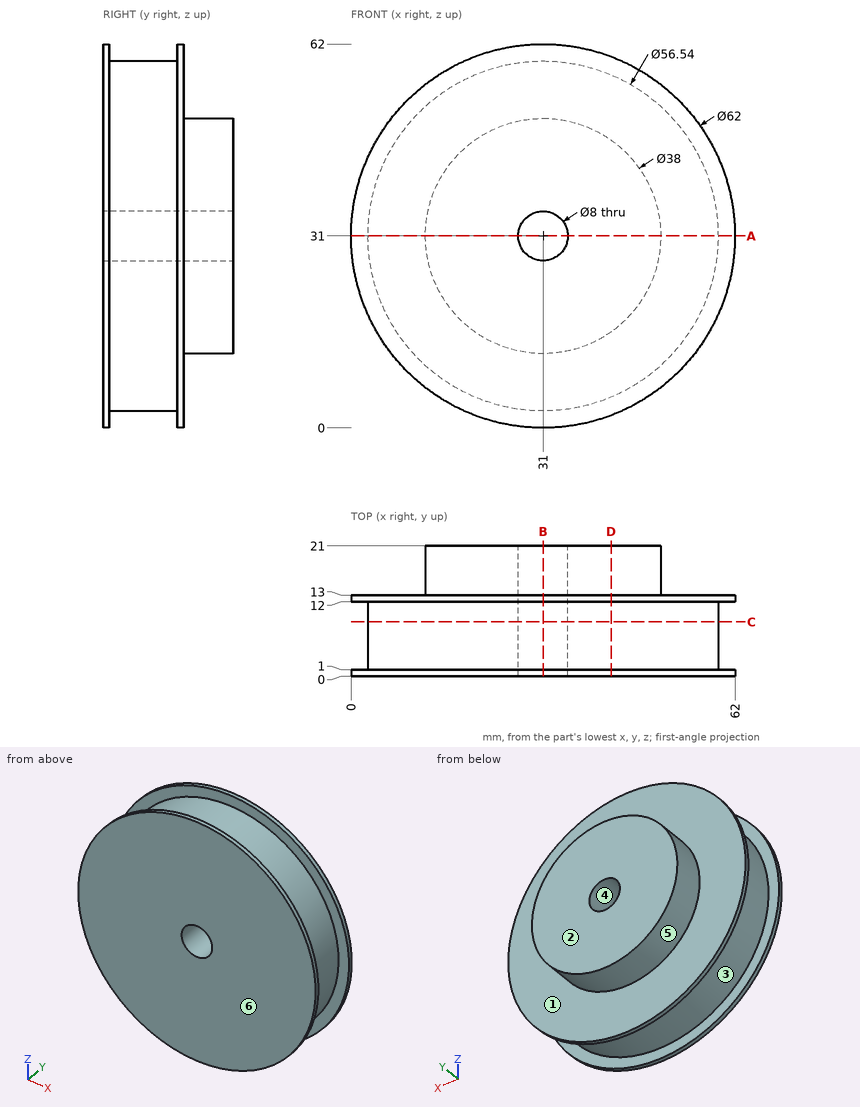
Job drawing, mm, ordinate dimensions from the low corner. One solid piece. A direction names the side the tool comes from. Give positions to 0.01 mm unless a question says otherwise; leave off trailing zeros. Loops run counter-clockwise (first coordinate to the right, second up) from the corner with the lowest first, then second, coordinate; pieces in that order, holes last. Notation, with made-up numbers: (-12.75, 59) - (10.25, 59) arc R19 cw to (10.25, 88) - close; hole circle Ø11 at (15, 2). An arc over 180 degrees is marked (long way). Use one line per item in the form item = value.
(1) 3-axis set-ups, long thin cutter, end or side, ignore diameter. For the marked faces 1, 2 and 3: which of +Z, -Z, +X, -X, +Y, -Y reach the whole face in a straight line?
Determined:
face_1 = +Y
face_2 = +Z, -Z, +X, -X, +Y
face_3 = none
(2) Cut at D-D (x = 42). Give the cut face in (y, z), then the cut area to 3 significant figures.
Determined:
outline = (0, 2.02) - (1, 2.02) - (1, 4.96) - (12, 4.96) - (12, 2.02) - (13, 2.02) - (13, 15.51) - (21, 15.51) - (21, 46.49) - (13, 46.49) - (13, 59.98) - (12, 59.98) - (12, 57.04) - (1, 57.04) - (1, 59.98) - (0, 59.98) - close
area = 937 mm^2
(3) Cut at B-B (x = 31). Give the cut face in (y, z), then the cut area to 3 significant figures.
Determined:
outline = (0, 0) - (1, 0) - (1, 2.73) - (12, 2.73) - (12, 0) - (13, 0) - (13, 12) - (21, 12) - (21, 27) - (0, 27) - close; (0, 35) - (21, 35) - (21, 50) - (13, 50) - (13, 62) - (12, 62) - (12, 59.27) - (1, 59.27) - (1, 62) - (0, 62) - close
area = 882 mm^2
(4) Pull direction X, two halves, no side cores. Call the marked faces 4, 5 and 6: pulls with the +X half, pulls with the -X half, needs draft (parallel to the pull), parting line crosses it, or undercut.
Determined:
face_4 = undercut
face_5 = parting line crosses it
face_6 = needs draft
(5) Cut at A-A (z = 31). Give the cut face in (x, y).
Determined:
outline = (0, 0) - (27, 0) - (27, 21) - (12, 21) - (12, 13) - (0, 13) - (0, 12) - (2.73, 12) - (2.73, 1) - (0, 1) - close; (35, 0) - (62, 0) - (62, 1) - (59.27, 1) - (59.27, 12) - (62, 12) - (62, 13) - (50, 13) - (50, 21) - (35, 21) - close
(6) Drop flat-ended pins along their axis: P1, Ø5, axis at y = 17, z = 23.5, coming from the -X side; P2, Ø2, axis at y = 15, z = 42.5, coming from the -X side; P3, Ø4, axis at x = 48, y = 11.5, coming from the -Z side. Give the stop position or say it passes through.
Determined:
P1 = 12.67
P2 = 15.16
P3 = 3.91
(7) Cut at C-C (y = 8.75). Give the cut face in (x, z).
Determined:
outline = circle Ø56.54 at (31, 31); hole circle Ø8 at (31, 31)
(8) Drill centre lines: L1, parallel to Y at x = 55, z = 47.5; L2, parallel to X at y = 14, z = 31; L3, parallel to X at y = 11.5, z = 31. Where is each one in solid material? Low to high.
Determined:
L1 = 0 to 1, 12 to 13
L2 = 12 to 27, 35 to 50
L3 = 2.73 to 27, 35 to 59.27
